For this review, use the dimensioned drawing (mm, ordinates from the lowest corner) and the shaded views. Round coordinates to 2 decimals unless told otherwise and drop trailing zeros. Write each loop counter-clockwise with the first axis right and the second up, starting at its lowest first coordinate (ties: lowest second). Pieces come first, ordered by that corner, then holes.
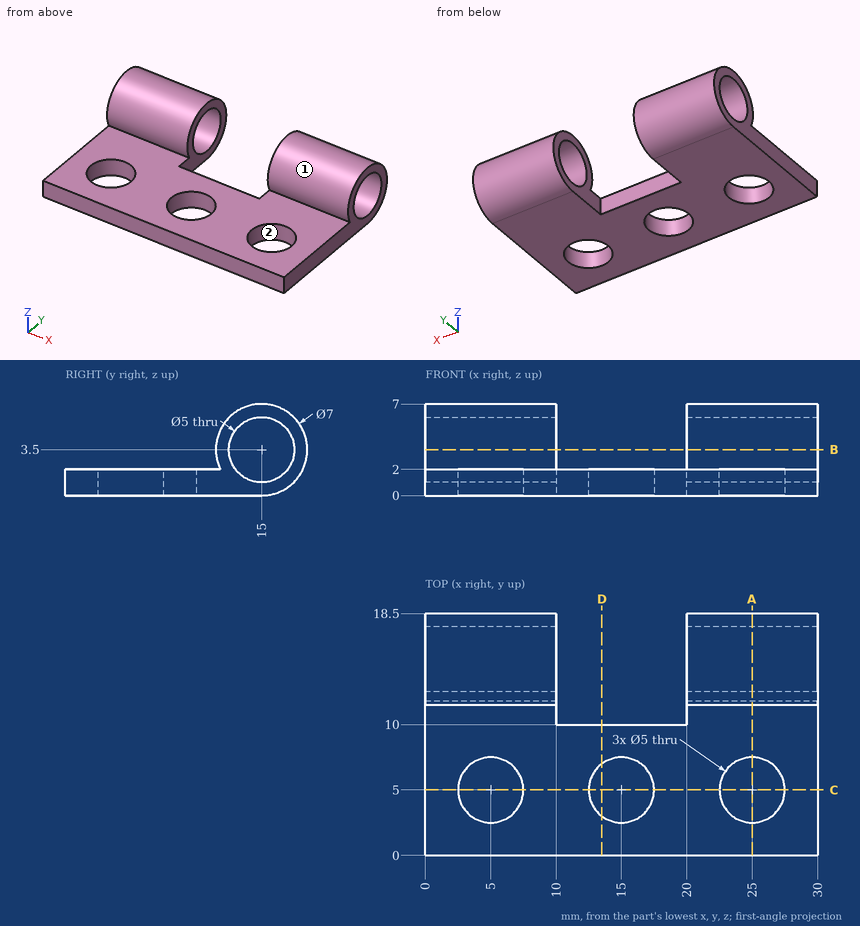
(1) For line 1 along Y through (x, z) = (4.5, 1.5); line 2 along Y through (x, z) = (2.5, 3.5); line 3 along X through (y, z) = (13.25, 1.25), list the stretches that pass through material, from the lowest coordinate up.
Geometry check:
line 1: y = 0 to 2.55, 7.45 to 13.5, 16.5 to 17.87
line 2: y = 11.5 to 12.5, 17.5 to 18.5
line 3: x = 0 to 10, 20 to 30
(2) We need section C-C, the plane y = 5. Give the boundary of the cut face in (x, z), and give its area (3 significant figures).
Geometry check:
outline: (0, 0) - (2.5, 0) - (2.5, 2) - (0, 2) - close; (7.5, 0) - (12.5, 0) - (12.5, 2) - (7.5, 2) - close; (17.5, 0) - (22.5, 0) - (22.5, 2) - (17.5, 2) - close; (27.5, 0) - (30, 0) - (30, 2) - (27.5, 2) - close
area: 30.0 mm2
(3) We need section B-B, the plane z = 3.5. Give the boundary of the cut face in (x, y).
Geometry check:
outline: (0, 11.5) - (10, 11.5) - (10, 12.5) - (0, 12.5) - close; (0, 17.5) - (10, 17.5) - (10, 18.5) - (0, 18.5) - close; (20, 11.5) - (30, 11.5) - (30, 12.5) - (20, 12.5) - close; (20, 17.5) - (30, 17.5) - (30, 18.5) - (20, 18.5) - close
(4) We need section A-A, the plane x = 25. Give the boundary of the cut face in (y, z), and give its area (3 significant figures).
Geometry check:
outline: (0, 0) - (2.5, 0) - (2.5, 2) - (0, 2) - close; (7.5, 0) - (15, 0) arc R3.5 ccw (long way) to (11.84, 2) - (7.5, 2) - close; hole circle Ø5 at (15, 3.5)
area: 34.3 mm2
(5) We need section D-D, the plane x = 13.5. Give the boundary of the cut face in (y, z).
Geometry check:
outline: (0, 0) - (3, 0) - (3, 2) - (0, 2) - close; (7, 0) - (10, 0) - (10, 2) - (7, 2) - close
(6) Mouldability with a two-part tool opening along X and no side actions: class the marked faces 1 and 2 as pulls with the +X half, pulls with the -X half, needs draft (parallel to the pull), parting line crosses it, or undercut.
Geometry check:
face 1: needs draft
face 2: undercut
(7) For pin 1 Ø3.5 at (x, y) = (10.5, 4) entering from +Z; pin 2 Ø2 at (x, z) = (12.5, 1.5) entering from +Y, all flat-tipped, find the tip position at first contact; note any pin that passes through.
Geometry check:
pin 1: stops at z = 2
pin 2: stops at y = 10
